```python
from build123d import *

# Parameters (mm, degrees)
F0_W      = 65
F0_H      = 60
F1_DEPTH  = 17.3
F3_START  = 25
F2_W      = 15.8
F2_H      = 13.3
F3_DEPTH  = 2.5
F5_D      = 5
F5_DEPTH  = 32.501
F2_W_2    = 8
F2_H_2    = 2.5
F6_DEPTH  = 30
F0_R      = 1.25
F7_DEPTH  = 2
F8_DEPTH  = 5
F9_DEPTH  = 17.3
F10_D     = 3
F10_DEPTH = 22
F10_TIP   = 0.9012909285
F11_DEPTH = 30
F12_R     = 5


# Not quite as in the source:
# - a feature names something its author has since deleted; it is built from what else it names


with BuildPart() as f1:
    # F0 (on Top) → F1 (new body)
    with BuildSketch(Plane.XY):
        Rectangle(F0_W, F0_H)
        with BuildLine():
            ThreePointArc((-30.5, 24.4646428929), (-30.517766953, 28.017766953), (-26.9646428929, 28))
            Line((-26.9646428929, 28), (26.9646428929, 28))
            ThreePointArc((26.9646428929, 28), (29.6951474044, 28.5644537982), (31.25, 26.25))
            ThreePointArc((31.25, 26.25), (31.0548861143, 25.2817541634), (30.5, 24.4646428929))
            Line((30.5, 24.4646428929), (30.5, -24.4646428929))
            ThreePointArc((30.5, -24.4646428929), (31.0548861143, -25.2817541634), (31.25, -26.25))
            ThreePointArc((31.25, -26.25), (29.6951474044, -28.5644537982), (26.9646428929, -28))
            Line((26.9646428929, -28), (-26.9646428929, -28))
            ThreePointArc((-26.9646428929, -28), (-30.517766953, -28.017766953), (-30.5, -24.4646428929))
            Line((-30.5, -24.4646428929), (-30.5, 24.4646428929))
        make_face(mode=Mode.SUBTRACT)
    extrude(amount=F1_DEPTH)

    # F2 (on Front) → F3 (cut)
    with BuildSketch(Plane.XZ.offset(F3_START)):
        with Locations((-8.7, 10.65)):
            Rectangle(F2_W, F2_H)
    extrude(amount=F3_DEPTH, mode=Mode.SUBTRACT)

    # F5 (through all, one way)
    with BuildSketch(Plane.YZ):
        with Locations((5, 15)):
            Circle(F5_D / 2)
    extrude(amount=-F5_DEPTH, mode=Mode.SUBTRACT)

    # F2 (on Front) → F6 (cut)
    with BuildSketch(Plane.XZ):
        with Locations((18.5, 5.25)):
            Rectangle(F2_W_2, F2_H_2)
    extrude(amount=F6_DEPTH, mode=Mode.SUBTRACT)

    # F0 (on Top) → F7 (join)
    with BuildSketch(Plane.XY):
        Rectangle(F0_W, F0_H)
        with BuildLine():
            ThreePointArc((-30.5, 24.4646428929), (-30.517766953, 28.017766953), (-26.9646428929, 28))
            Line((-26.9646428929, 28), (26.9646428929, 28))
            ThreePointArc((26.9646428929, 28), (29.6951474044, 28.5644537982), (31.25, 26.25))
            ThreePointArc((31.25, 26.25), (31.0548861143, 25.2817541634), (30.5, 24.4646428929))
            Line((30.5, 24.4646428929), (30.5, -24.4646428929))
            ThreePointArc((30.5, -24.4646428929), (31.0548861143, -25.2817541634), (31.25, -26.25))
            ThreePointArc((31.25, -26.25), (29.6951474044, -28.5644537982), (26.9646428929, -28))
            Line((26.9646428929, -28), (-26.9646428929, -28))
            ThreePointArc((-26.9646428929, -28), (-30.517766953, -28.017766953), (-30.5, -24.4646428929))
            Line((-30.5, -24.4646428929), (-30.5, 24.4646428929))
        make_face(mode=Mode.SUBTRACT)
        with BuildLine():
            Line((26.9646428929, 28), (-26.9646428929, 28))
            ThreePointArc((-26.9646428929, 28), (-26.4355462018, 27.1951474044), (-26.25, 26.25))
            ThreePointArc((-26.25, 26.25), (-27.7817541634, 23.9451138857), (-30.5, 24.4646428929))
            Line((-30.5, 24.4646428929), (-30.5, -24.4646428929))
            ThreePointArc((-30.5, -24.4646428929), (-27.7817541634, -23.9451138857), (-26.25, -26.25))
            ThreePointArc((-26.25, -26.25), (-26.4355462018, -27.1951474044), (-26.9646428929, -28))
            Line((-26.9646428929, -28), (26.9646428929, -28))
            ThreePointArc((26.9646428929, -28), (26.982233047, -24.482233047), (30.5, -24.4646428929))
            Line((30.5, -24.4646428929), (30.5, 24.4646428929))
            ThreePointArc((30.5, 24.4646428929), (26.982233047, 24.482233047), (26.9646428929, 28))
        make_face()
        with Locations((-22.5, -24)):
            Circle(F0_R, mode=Mode.SUBTRACT)
        with Locations((4.5, -24)):
            Circle(F0_R, mode=Mode.SUBTRACT)
        with Locations((13.95, -20)):
            Circle(F0_R, mode=Mode.SUBTRACT)
        with Locations((22.5, -20)):
            Circle(F0_R, mode=Mode.SUBTRACT)
        with BuildLine():
            Line((-26.9646428929, 28), (-30.5, 28))
            Line((-30.5, 28), (-30.5, 24.4646428929))
            ThreePointArc((-30.5, 24.4646428929), (-27.7817541634, 23.9451138857), (-26.25, 26.25))
            ThreePointArc((-26.25, 26.25), (-26.4355462018, 27.1951474044), (-26.9646428929, 28))
        make_face()
        with BuildLine():
            Line((30.5, 28), (26.9646428929, 28))
            ThreePointArc((26.9646428929, 28), (26.982233047, 24.482233047), (30.5, 24.4646428929))
            Line((30.5, 24.4646428929), (30.5, 28))
        make_face()
        with BuildLine():
            ThreePointArc((-26.25, -26.25), (-27.7817541634, -23.9451138857), (-30.5, -24.4646428929))
            Line((-30.5, -24.4646428929), (-30.5, -28))
            Line((-30.5, -28), (-26.9646428929, -28))
            ThreePointArc((-26.9646428929, -28), (-26.4355462018, -27.1951474044), (-26.25, -26.25))
        make_face()
        with BuildLine():
            Line((30.5, -28), (30.5, -24.4646428929))
            ThreePointArc((30.5, -24.4646428929), (26.982233047, -24.482233047), (26.9646428929, -28))
            Line((26.9646428929, -28), (30.5, -28))
        make_face()
        with Locations((22.5, -20)):
            Circle(F0_R)
        with Locations((13.95, -20)):
            Circle(F0_R)
        with Locations((-22.5, -24)):
            Circle(F0_R)
        with Locations((4.5, -24)):
            Circle(F0_R)
        with BuildLine():
            Line((-30.5, 24.4646428929), (-30.5, 28))
            Line((-30.5, 28), (-26.9646428929, 28))
            ThreePointArc((-26.9646428929, 28), (-30.517766953, 28.017766953), (-30.5, 24.4646428929))
        make_face()
        with BuildLine():
            ThreePointArc((31.25, 26.25), (29.6951474044, 28.5644537982), (26.9646428929, 28))
            Line((26.9646428929, 28), (30.5, 28))
            Line((30.5, 28), (30.5, 24.4646428929))
            ThreePointArc((30.5, 24.4646428929), (31.0548861143, 25.2817541634), (31.25, 26.25))
        make_face()
        with BuildLine():
            Line((-30.5, -28), (-30.5, -24.4646428929))
            ThreePointArc((-30.5, -24.4646428929), (-30.517766953, -28.017766953), (-26.9646428929, -28))
            Line((-26.9646428929, -28), (-30.5, -28))
        make_face()
        with BuildLine():
            ThreePointArc((31.25, -26.25), (31.0548861143, -25.2817541634), (30.5, -24.4646428929))
            Line((30.5, -24.4646428929), (30.5, -28))
            Line((30.5, -28), (26.9646428929, -28))
            ThreePointArc((26.9646428929, -28), (29.6951474044, -28.5644537982), (31.25, -26.25))
        make_face()
    extrude(amount=-F7_DEPTH)

    # F0 (on Top) → F8 (join)
    with BuildSketch(Plane.XY):
        with Locations((22.5, -20)):
            Circle(F0_R)
        with Locations((13.95, -20)):
            Circle(F0_R)
        with Locations((-22.5, -24)):
            Circle(F0_R)
        with Locations((4.5, -24)):
            Circle(F0_R)
    extrude(amount=F8_DEPTH)

    # F0 (on Top) → F9 (join)
    with BuildSketch(Plane.XY):
        with BuildLine():
            Line((30.5, -28), (30.5, -24.4646428929))
            ThreePointArc((30.5, -24.4646428929), (26.982233047, -24.482233047), (26.9646428929, -28))
            Line((26.9646428929, -28), (30.5, -28))
        make_face()
        with BuildLine():
            ThreePointArc((31.25, -26.25), (31.0548861143, -25.2817541634), (30.5, -24.4646428929))
            Line((30.5, -24.4646428929), (30.5, -28))
            Line((30.5, -28), (26.9646428929, -28))
            ThreePointArc((26.9646428929, -28), (29.6951474044, -28.5644537982), (31.25, -26.25))
        make_face()
        with BuildLine():
            ThreePointArc((31.25, 26.25), (29.6951474044, 28.5644537982), (26.9646428929, 28))
            Line((26.9646428929, 28), (30.5, 28))
            Line((30.5, 28), (30.5, 24.4646428929))
            ThreePointArc((30.5, 24.4646428929), (31.0548861143, 25.2817541634), (31.25, 26.25))
        make_face()
        with BuildLine():
            Line((30.5, 28), (26.9646428929, 28))
            ThreePointArc((26.9646428929, 28), (26.982233047, 24.482233047), (30.5, 24.4646428929))
            Line((30.5, 24.4646428929), (30.5, 28))
        make_face()
        with BuildLine():
            Line((-26.9646428929, 28), (-30.5, 28))
            Line((-30.5, 28), (-30.5, 24.4646428929))
            ThreePointArc((-30.5, 24.4646428929), (-27.7817541634, 23.9451138857), (-26.25, 26.25))
            ThreePointArc((-26.25, 26.25), (-26.4355462018, 27.1951474044), (-26.9646428929, 28))
        make_face()
        with BuildLine():
            Line((-30.5, 24.4646428929), (-30.5, 28))
            Line((-30.5, 28), (-26.9646428929, 28))
            ThreePointArc((-26.9646428929, 28), (-30.517766953, 28.017766953), (-30.5, 24.4646428929))
        make_face()
        with BuildLine():
            Line((-30.5, -28), (-30.5, -24.4646428929))
            ThreePointArc((-30.5, -24.4646428929), (-30.517766953, -28.017766953), (-26.9646428929, -28))
            Line((-26.9646428929, -28), (-30.5, -28))
        make_face()
        with BuildLine():
            ThreePointArc((-26.25, -26.25), (-27.7817541634, -23.9451138857), (-30.5, -24.4646428929))
            Line((-30.5, -24.4646428929), (-30.5, -28))
            Line((-30.5, -28), (-26.9646428929, -28))
            ThreePointArc((-26.9646428929, -28), (-26.4355462018, -27.1951474044), (-26.25, -26.25))
        make_face()
    extrude(amount=F9_DEPTH)

    # F10 (one way)
    with BuildSketch(Plane(origin=(0, 0, 0), x_dir=(1, 0, 0), z_dir=(0, 0, -1))):
        with Locations((-28.75, -26.25), (28.75, -26.25), (28.75, 26.25), (-28.75, 26.25)):
            Circle(F10_D / 2)
    extrude(amount=-F10_DEPTH, mode=Mode.SUBTRACT)
    with Locations(Plane(origin=(0, 0, 0), x_dir=(1, 0, 0), z_dir=(0, 0, -1))):
        with Locations((-28.75, -26.25), (28.75, -26.25), (28.75, 26.25), (-28.75, 26.25)):
            with Locations((0, 0, -(F10_DEPTH + F10_TIP / 2))):  # 118° drill point
                Cone(0, F10_D / 2, F10_TIP, mode=Mode.SUBTRACT)

    # F2 (on Front) → F11 (cut)
    with BuildSketch(Plane.XZ):
        with Locations((-8.7, 10.65)):
            Rectangle(F2_W, F2_H)
    extrude(amount=F11_DEPTH, mode=Mode.SUBTRACT)

    # F12
    f12_edges = [f1.edges().sort_by_distance(p)[0] for p in [
        (32.5, -30, 7.65),
        (32.5, 30, 7.65),
        (-32.5, 30, 7.65),
        (-32.5, -30, 7.65),
    ]]
    fillet(f12_edges, radius=F12_R)


solid = f1.part
```
Input: part model. Units: mm. Frame: model coordinates. A direction names the side the tool comes from. Round coordinates to 2 decimals unless told otherwise and drop trailing zeros. Loops run counter-clockwise (first coordinate to the right, second up) from the corner with the lowest first, then second, coordinate; pieces in that order, holes last. Notation, with made-up numbers: M 48,54.5 L 91,54.5 A9 cw 91,65.5 Z; hole C 84,67 d11. An arc over 180 degrees is marked long. Answer in a Markdown table with one row per item. Add a question column.
1. Set-up query: faces 4 (the face through (22, -20, 5)), 5 (the face through (31.07, -28.5, 7.79)), 6 (the face through (-9, -29, 4)), 7 (the face through (18, -29, 6.5)), 8 (the face through (31, 28.57, 7.51)). Return all of +Z, -Z, +X, -X, +Y, -Y with unobstructed straight access to the full face (end or side cutting, diameter ignored); none if empty.
2. Ray query, probe 1 along X at (y, z) = (21.5, 3.25); probe 2 along X at (y, z) = (26.5, 5.75); probe 3 along Y at (x, z) = (28.5, 12.5). Return the intervals inside material, ascending.
3. Section C-C (z = 11.5). Output: boundary loops of the cut face in (x, y), and give its area (3 significant figures).
4. Contact query for flat-ended pins moving along their axis: pin 1 (1 mm diameter, centred on y = -28.5, z = 7.5, fed in from -X); pin 2 (4 mm diameter, centred on x = 8, y = 12.5, fed in from +Z); pin 3 (1.2 mm diameter, centred on x = 23, y = -20, fed in from +Z). Output: stop coordinate, or through.
5. Mould query, pull axis X, two halves, no side actions, for faces 1 (the face through (-31.07, -28.5, 7.79)), 2 (the face through (15.105, -20.479, 2.465)), 3 (the face through (0, 0, -2)). Classes: released by +X, released by -X, zero draft, split by the parting line, or undercut.
6. Section B-B (y = -8). Output: boundary loops of the cut face in (x, z).
7. Section A-A (z = 15). Output: boundary loops of the cut face in (x, y), and give its area (3 significant figures).
8. Section D-D (x = 4.5). Output: boundary loops of the cut face in (y, z), and give its area (3 significant figures).
Values follow:
| question | item | result |
|---|---|---|
| 1 | face 4 | +Z |
| 1 | face 5 | +Z, -Z, +X, -Y |
| 1 | face 6 | +Z, -Y |
| 1 | face 7 | -Y |
| 1 | face 8 | +Z, -Z, +X, +Y |
| 2 | probe 1 | -32.5 to -30.5, 30.5 to 32.5 |
| 2 | probe 2 | -32.27 to -30.23, -27.27 to -26.26, 26.26 to 27.27, 30.23 to 32.27 |
| 2 | probe 3 | -29.9 to -27.73, -24.77 to -23.76, 23.76 to 24.77, 27.73 to 29.9 |
| 3 | outline | M -32.5,-25 A5 ccw -27.5,-30 L -16.6,-30 L -16.6,-28 L -26.96,-28 A2.5 ccw -30.5,-24.46 L -30.5,24.46 A2.5 ccw -26.96,28 L 26.96,28 A2.5 ccw 30.5,24.46 L 30.5,-24.46 A2.5 ccw 26.96,-28 L -0.8,-28 L -0.8,-30 L 27.5,-30 A5 ccw 32.5,-25 L 32.5,25 A5 ccw 27.5,30 L -27.5,30 A5 ccw -32.5,25 Z; hole C -28.75,-26.25 d3; hole C -28.75,26.25 d3; hole C 28.75,-26.25 d3; hole C 28.75,26.25 d3 |
| 3 | area | 466 mm^2 |
| 4 | pin 1 | x = -31.5 |
| 4 | pin 2 | z = 0 |
| 4 | pin 3 | z = 5 |
| 5 | face 1 | released by -X |
| 5 | face 2 | undercut |
| 5 | face 3 | zero draft |
| 6 | outline | M -32.5,-2 L 32.5,-2 L 32.5,17.3 L 30.5,17.3 L 30.5,0 L -30.5,0 L -30.5,17.3 L -32.5,17.3 Z |
| 7 | outline | M -32.5,-25 A5 ccw -27.5,-30 L -16.6,-30 L -16.6,-28 L -26.96,-28 A2.5 ccw -30.5,-24.46 L -30.5,2.5 L -32.5,2.5 Z; M -32.5,7.5 L -30.5,7.5 L -30.5,24.46 A2.5 ccw -26.96,28 L 26.96,28 A2.5 ccw 30.5,24.46 L 30.5,-24.46 A2.5 ccw 26.96,-28 L -0.8,-28 L -0.8,-30 L 27.5,-30 A5 ccw 32.5,-25 L 32.5,25 A5 ccw 27.5,30 L -27.5,30 A5 ccw -32.5,25 Z; hole C -28.75,-26.25 d3; hole C -28.75,26.25 d3; hole C 28.75,-26.25 d3; hole C 28.75,26.25 d3 |
| 7 | area | 456 mm^2 |
| 8 | outline | M -30,-2 L 30,-2 L 30,17.3 L 28,17.3 L 28,0 L -22.75,0 L -22.75,5 L -25.25,5 L -25.25,0 L -28,0 L -28,17.3 L -30,17.3 Z |
| 8 | area | 202 mm^2 |
